Autodesk Inventor part; units mm, degrees
ref_plane "YZ Plane" through (0, 0, 0) normal (1, 0, 0) x (0, 1, 0)
ref_plane "XZ Plane" through (0, 0, 0) normal (0, 1, 0) x (-1, 0, 0)
ref_plane "XY Plane" through (0, 0, 0) normal (0, 0, 1) x (1, 0, 0)
sketch "Sketch1" plane through (0, 0, 0) normal (0, 1, 0) x (-1, 0, 0)
  line L0 (-12, 95) -> (-12, 5)
  line L1 (-12, 5) -> (-12, 95)
  line L2 (-7, 100) -> (76.1843, 100)
  line L3 (76.1843, 100) -> (-7, 100)
  line L4 (76.0718, 100) -> (83, 100)
  line L5 (-7, 100) -> (83, 100)
  line L6 (88, 11.9282) -> (88, 5)
  line L7 (88, 95) -> (88, 5)
  line L8 (-0.0718, 0) -> (-7, 0)
  line L9 (-7, 0) -> (83, 0)
  arc A0 (-12, 5) -> (-7, 0) centre (-7, 5) ccw
  arc A1 (-7, 100) -> (-12, 95) centre (-7, 95) ccw
  line L10 (88, 5) -> (88, 95)
  arc A2 (88, 95) -> (83, 100) centre (83, 95) ccw
  arc A3 (83, 0) -> (88, 5) centre (83, 5) ccw
  arc A4 (-12, 5) -> (-7, 0) centre (-7, 5) ccw
  circle A5 centre (-7, 5) radius 1.5
  circle A6 centre (-7, 95) radius 1.5
  circle A7 centre (83, 95) radius 1.5
  circle A8 centre (83, 5) radius 1.5
  line L11 (88, 17.761) -> (79.7328, 17.761)
  line L12 (79.7328, 17.761) -> (79.7328, 28.761)
  line L13 (79.7328, 28.761) -> (88, 28.761)
  line L14 (88, 28.761) -> (88, 17.761)
extrude "Extrusion1" add sketch "Sketch1" against normal blind 3 contours A1 L2 L4 A2 L7 L13 L12 L11 L6 A3 L9 L8 A0 L0
extrude "Extrusion2" add sketch "Sketch1" against normal blind 3.2 contours L7 L11 L12 L13
sketch "PiHoles" plane through (0, -3, 0) normal (0, -1, 0) x (1, 0, 0)
  line L0 (-79.7328, 28.761) -> (-79.7328, 17.761)
  line L1 (-88, 5) -> (-88, 95)
  circle A0 centre (-76, 15.761) radius 1.25
  circle A1 centre (-76, 15.761) radius 3
  circle A2 centre (-76, 73.761) radius 1.25
  circle A3 centre (-76, 73.761) radius 3
  circle A4 centre (-53, 15.761) radius 1.25
  circle A5 centre (-53, 15.761) radius 3
  circle A6 centre (-53, 73.761) radius 1.25
  circle A7 centre (-53, 73.761) radius 3
  circle A8 centre (-53, 73.761) radius 0.75
  circle A9 centre (-53, 15.761) radius 0.75
  circle A10 centre (-76, 73.761) radius 0.75
  circle A11 centre (-76, 15.761) radius 0.75
  circle A12 centre (-41.4372, 81.0897) radius 1.25
  circle A13 centre (-41.4372, 81.0897) radius 3
  circle A14 centre (-41.4372, 81.0897) radius 0.75
  circle A15 centre (-41.4178, 92.9645) radius 0.75
  circle A16 centre (-41.4178, 92.9645) radius 1.25
  circle A17 centre (-41.4178, 92.9645) radius 3
  circle A18 centre (-32.9361, 81.2633) radius 0.75
  circle A19 centre (-32.9361, 81.2633) radius 1.25
  circle A20 centre (-32.9361, 81.2633) radius 2
  circle A21 centre (-32.9166, 93.1381) radius 0.75
  circle A22 centre (-32.9166, 93.1381) radius 1.25
  circle A23 centre (-32.9166, 93.1381) radius 1.75
  point P0 (-79.7328, 23.261)
  point P1 (-88, 23.261)
  point P2 (-76, 23.261)
  point P3 (-76, 23.261)
  point P4 (-52, 74.761)
  point P5 (-41.4372, 93.09)
  point P6 (-40.4372, 94.09)
  dimension "d4" = 2.5
  dimension "d5" = 6
  dimension "d6" = 2.5
  dimension "d7" = 6
  dimension "d8" = 2.5
  dimension "d9" = 6
  dimension "d10" = 2.5
  dimension "d11" = 6
  dimension "d21" = 1.5
  dimension "d22" = 1.5
  dimension "d23" = 1.5
  dimension "d24" = 1.5
  dimension "d30" = 2.5
  dimension "d31" = 6
  dimension "d32" = 1.5
  dimension "d33" = 2.5
  dimension "d34" = 6
  dimension "d35" = 1.5
  dimension "d40" = 2.5
  dimension "d41" = 4
  dimension "d42" = 1.5
  dimension "d43" = 2.5
  dimension "d44" = 3.5
  dimension "d45" = 1.5
extrude "Extrusion3" add sketch "PiHoles" along normal blind 3 contours A1 | A3 | A5 | A7
extrude "Extrusion4" cut sketch "PiHoles" against normal blind 2 contours A8 | A9 | A10 | A11
extrude "Extrusion5" add sketch "PiHoles" along normal blind 2 contours A13 | A17
extrude "Extrusion6" cut sketch "PiHoles" against normal blind 2 contours A14 | A15
extrude "Extrusion7" add sketch "PiHoles" along normal blind 2 contours A20 | A23
properties part number "groundplate"
Source: CAD feature listing. Evaluate the final solid. Frame: model axes, mm. A direction names the side the tool comes from. Give positions to 0.01 mm unless a question says otherwise; leave off trailing zeros. Write each loop counter-clockwise with the first axis right and the second up, starting at its lowest first coordinate (ties: lowest second). Pieces come first, ordered by that corner, then holes.
1. First-contact query: pin 1 (1.5 mm diameter, centred on x = -32.94, z = 81.26, fed in from -Y); pin 2 (0.8 mm diameter, centred on x = -76, z = 73.5, fed in from -Y); pin 3 (3 mm diameter, centred on x = -41.42, z = 92.96, fed in from -Y); pin 4 (1 mm diameter, centred on y = -4, z = 56.5, fed in from +X). Flat tips, straight axial feed; report the tip coordinate or a pass-through.
2. Section query B-B (z = 37.5). Return the cut outline in (x, y).
3. Access query for faces 1 (the face through (-75.42, -4.48, 74.87)), 2 (the face through (-37, -1, 0)). Directions: +Z, -Z, +X, -X, +Y, -Y. A direction counts if a zero-diameter tool reaches every point of the face in a straight line with its end or side. Return the directions, or none.
4. Section query A-A (x = -68.5). Return the cut outline in (y, z), then the cut area to 3 significant figures.
5. Material intervals for line 1 along Z through (x, y) = (-76, -1.8); line 2 along X through (y, z) = (-0.65, 95); line 3 along Z through (x, y) = (-76, -4.6), sorted ascending.
6. Pull-direction query (X, two-part tool) for faces 3 (the face through (-55.997, -4.479, 15.629)), 4 (the face through (8.5, -1.48, 5.07)), 5 (the face through (-76, -6, 14)); classes: +X half, -X half, draft (parallel to the pull), parting line (faces both ways), or undercut.
Output values:
1. pin 1: stops at y = -3
1. pin 2: stops at y = -1
1. pin 3: stops at y = -5
1. pin 4: passes through
2. outline: (-88, -3) - (12, -3) - (12, 0) - (-88, 0) - close
3. face 1: -Y
3. face 2: -Z, +X, -X, +Y, -Y
4. outline: (-3, 0) - (0, 0) - (0, 100) - (-3, 100) - close
4. area: 300 mm2
5. line 1: z = 0 to 15.01, 16.51 to 73.01, 74.51 to 100
5. line 2: x = -88 to -84.5, -81.5 to 5.5, 8.5 to 12
5. line 3: z = 12.76 to 14.51, 17.01 to 18.76, 70.76 to 72.51, 75.01 to 76.76
6. face 3: undercut
6. face 4: undercut
6. face 5: draft
